Autodesk Inventor part; units mm, degrees
ref_plane "YZ Plane" through (0, 0, 0) normal (1, 0, 0) x (0, 1, 0)
ref_plane "XZ Plane" through (0, 0, 0) normal (0, 1, 0) x (-1, 0, 0)
ref_plane "XY Plane" through (0, 0, 0) normal (0, 0, 1) x (1, 0, 0)
sketch "スケッチ1" plane through (0, 0, 0) normal (0, 0, 1) x (1, 0, 0)
  line L0 (-20, -2.5) -> (20, -2.5)
  line L1 (20, -2.5) -> (20, 2.5)
  line L2 (-20, 2.5) -> (-20, -2.5)
  line L3 (-20, -2.5) -> (20, 2.5) construction
  line L4 (20, -2.5) -> (-20, 2.5) construction
  line L5 (-10, 2.5) -> (10, 2.5)
  line L6 (10, 2.5) -> (10, 53.5)
  line L7 (10, 53.5) -> (-10, 53.5)
  line L8 (-10, 53.5) -> (-10, 2.5)
  line L9 (-10, 2.5) -> (10, 53.5) construction
  line L10 (10, 2.5) -> (-10, 53.5) construction
  line L11 (20, 2.5) -> (10, 2.5)
  line L12 (-10, 2.5) -> (-20, 2.5)
  line L13 (0, 53.5) -> (0, -2.5)
  point P0 (0, 0)
  point P1 (0, 28)
  point P2 (0, 28)
  point P3 (0, 0)
  dimension "d0" = 20
  dimension "d1" = 51
  dimension "d2" = 5
  dimension "d3" = 10
extrude "押し出し1" add sketch "スケッチ1" along normal mid plane 210 contours L13 L5 L11 L1 L0 | L13 L7 L6 L5
sketch "スケッチ4" plane through (0, -2.5, 105) normal (-1, 0, 0) x (0, 0, 1)
  line L0 (0, 7) -> (-34.3102, 56)
  line L1 (-210, 56) -> (0, 56)
  line L2 (0, 56) -> (0, 0)
  line L3 (0, 5) -> (-210, 5)
  point P0 (-105, 2.5)
  dimension "d18" = 35
  dimension "d21" = 2
extrude "押し出し3" cut sketch "スケッチ4" against normal through all
sketch "スケッチ5" plane through (10, 2.5, -105) normal (1, 0, 0) x (0, 0, -1)
  circle A0 centre (-158, 44) radius 6.05
  line L0 (0, 0) -> (-210, 0)
  line L1 (-210, 0) -> (-210, 2)
  point P0 (-105, -2.5)
  dimension "d22" = 12.1
  dimension "d23" = 44
  dimension "d37" = 52
extrude "押し出し4" cut sketch "スケッチ5" against normal blind 10
sketch "スケッチ6" plane through (10, 2.5, 105) normal (0, 1, 0) x (1, 0, 0)
  line L0 (10, 210) -> (10, 0)
  line L1 (10, 0) -> (0, 0)
  line L2 (0, 210) -> (10, 210)
  point P0 (-10, 105)
  point P1 (5, 205)
  point P2 (5, 5)
  point P3 (5, 60)
  point P4 (5, 95)
  dimension "d27" = 5
  dimension "d28" = 5
  dimension "d29" = 5
  dimension "d50" = 35
  dimension "d51" = 55
hole "穴2" at (15, 2.5, -100) at (15, 2.5, 100) at (15, 2.5, 45) at (15, 2.5, 10) direction (0, -1, 0) diameter 3.4 end through all
sketch "スケッチ9" plane through (10, -2.5, -105) normal (-1, 0, 0) x (0, 0, 1)
  circle A0 centre (158, 49) radius 6.05
  line L0 (139.4081, 15.2287) -> (179.2189, 43.1045)
  line L1 (179.2189, 43.1045) -> (159.7173, 70.9557)
  line L2 (159.7173, 70.9557) -> (119.9065, 43.0798)
  line L3 (119.9065, 43.0798) -> (139.4081, 15.2287)
  line L4 (139.4081, 15.2287) -> (159.7173, 70.9557) construction
  line L5 (179.2189, 43.1045) -> (119.9065, 43.0798) construction
  line L6 (210, 7) -> (175.6898, 56)
  line L7 (158, 49) -> (149.5627, 43.0922) construction
  point P0 (157.2238, 55)
  point P1 (158.7762, 55)
  dimension "d123" = 48.6
  dimension "d124" = 34
  dimension "d125" = 14
hole "穴6" at (10, 40.5798, 14.9065) at (10, 12.7287, 34.4081) at (10, 40.6045, 74.2189) direction (-1, 0, 0) diameter 4.5 end through all counterbore diameter 8 counterbore depth 4
sketch "スケッチ14" plane through (10, 2.5, -105) normal (1, 0, 0) x (0, 0, -1)
  line L0 (0, 51) -> (0, 0)
  line L1 (0, 51) -> (-175.6898, 51)
  line L2 (0, 0) -> (-210, 0)
  line L3 (-175.6898, 51) -> (-210, 2)
  point P0 (-105, -2.5)
  point P1 (-173.087, 46)
  point P2 (-200.3951, 7)
  point P3 (-5, 46)
  point P4 (-5, 7)
  dimension "d126" = 5
  dimension "d127" = 5
  dimension "d128" = 7
  dimension "d129" = 5
  dimension "d130" = 5
hole "穴9" at (10, 48.5, 68.087) at (10, 9.5, 95.3951) at (10, 48.5, -100) at (10, 9.5, -100) direction (-1, 0, 0) diameter 3.4 end through all counterbore diameter 6.5 counterbore depth 4
fillet "フィレット1" radius 5 2 edges at (5, 53.5, -105) (5, 53.5, 70.6898)
properties part number "s_base4" material "ABS プラスチック"
The model under review builds one solid part; all positions refer to its coordinate system, in mm. A direction names the side the tool comes from. Round coordinates to 2 decimals unless told otherwise and drop trailing zeros. Write each loop counter-clockwise with the first axis right and the second up, starting at its lowest first coordinate (ties: lowest second). Pieces come first, ordered by that corner, then holes. Notation, with made-up numbers: (13, 35.25) - (37, 35.25) arc R14 ccw to (37, 43.25) - close; hole circle Ø6 at (44, 9.25). An arc over 180 degrees is marked (long way). Use one line per item in the form item = value.
Q1. Insertion check: pin 1 Ø2.5 at (y, z) = (11, 35.5) entering from +X; pin 2 Ø6 at (x, z) = (15, -76) entering from +Y; pin 3 Ø12 at (x, y) = (3, 36.5) entering from +Z. Each pin has a flat end and moves straight along its axis. Give the tip position at first contact, or say it passes through.
Answer key:
pin_1 = 6
pin_2 = 2.5
pin_3 = 86.79
Q2. Consider section B-B (y = 23). State the section outline as (x, z) points, and give its area (3 significant figures).
Answer key:
outline = (0, -105) - (10, -105) - (10, 92.05) - (0, 92.05) - close
area = 1,970 mm2
Q3. Consider section A-A (z = 28.5). State the section outline as (x, y) points, and give its area (3 significant figures).
Answer key:
outline = (0, -2.5) - (20, -2.5) - (20, 2.5) - (10, 2.5) - (10, 53.5) - (0, 53.5) - close
area = 610 mm2
Q4. For line 1 (Z direction, x = 15, y = 0.95); line 2 (Z direction, x = 1.2, y = 48.5); line 3 (Z direction, x = 8, y = 49), list the stretches that pass through material, from the lowest coordinate up. Write a range as [from, to].
Answer key:
line_1 = [-105, -101.7], [-98.3, 8.3], [11.7, 43.3], [46.7, 98.3], [101.7, 105]
line_2 = [-105, -101.7], [-98.3, 47.29], [58.71, 66.39], [69.79, 74.19]
line_3 = [-104.97, -103.21], [-96.79, 47.49], [58.51, 64.88], [71.3, 73.84]
Q5. Draft analysis for pull direction Y (two halves, no side actions). For faces 1 (the cylindrical face through (4.93, 52.07, -103.5)), 2 (the cylindrical face through (14.93, -0.04, -101.7)), 3 (the cylindrical face through (7.972, 8.524, 92.295)), state which applies: +Y half, -Y half, draft (parallel to the pull), parting line (faces both ways), or undercut.
Answer key:
face_1 = +Y half
face_2 = draft
face_3 = undercut
Q6. Tool access review of faces 4 (the flat face through (6, 42, 72)), 5 (the cylindrical face through (2.958, 49.151, 66.517)): name each direction out of +Z, -Z, +X, -X, +Y, -Y from which nothing blocks a thin tool from reaching the whole face with its end or side.
Answer key:
face_4 = +X
face_5 = +X, -X
